```python
from build123d import *

# Parameters (mm, degrees)
SKETCH_1_R               = 11.5
EXTRUDE_1_DEPTH          = 10
SKETCH_2_R               = 13.945
EXTRUDE_2_DEPTH          = 13
SKETCH_3_R               = 16
EXTRUDE_3_DEPTH          = 1
EXTRUDE_START            = -1
SKETCH_4_R               = 16
EXTRUDE_4_DEPTH          = 1
CUT_EXTRUDE_1_DEPTH      = 33.26453161
CUT_EXTRUDE_1_DEPTH_BACK = 33.26453161
SKETCH_5_R               = 2.5


with BuildPart() as part:
    # 草图1 → 凸台-拉伸1 (new body)
    with BuildSketch(Plane.XY):
        Circle(SKETCH_1_R)
    extrude(amount=-EXTRUDE_1_DEPTH)

    # 草图2 → 凸台-拉伸2 (add)
    with BuildSketch(Plane(origin=(0, 0, -10), x_dir=(-1, 0, 0), z_dir=(0, 0, -1))):
        with Locations(Location((0, 0, 0), (0, 0, 180))):
            Circle(SKETCH_2_R)
    extrude(amount=EXTRUDE_2_DEPTH)

    # 草图3 → 凸台-拉伸3 (add)
    with BuildSketch(Plane(origin=(0, 0, -23), x_dir=(-1, 0, 0), z_dir=(0, 0, -1))):
        Circle(SKETCH_3_R)
    extrude(amount=-EXTRUDE_3_DEPTH)

    # 草图4 → 凸台-拉伸4 (add)
    with BuildSketch(Plane.XY.offset(-10).offset(EXTRUDE_START)):
        with Locations(Location((0, 0, 0), (0, 0, 180))):
            Circle(SKETCH_4_R)
    extrude(amount=EXTRUDE_4_DEPTH)

    # 草图5 → 切除-拉伸1 (cut, two sides: drawn at the far end of the back side and taken through both)
    with BuildSketch(Plane.XY.offset(-CUT_EXTRUDE_1_DEPTH_BACK)):
        Circle(SKETCH_5_R)
    extrude(amount=CUT_EXTRUDE_1_DEPTH + CUT_EXTRUDE_1_DEPTH_BACK, mode=Mode.SUBTRACT)


solid = part.part
```
The model under review builds one solid part; all positions refer to its coordinate system, in mm. A direction names the side the tool comes from. Coordinates: 2 decimals unless noted, no trailing zeros. Write each loop counter-clockwise with the first axis right and the second up, starting at its lowest first coordinate (ties: lowest second). Pieces come first, ordered by that corner, then holes. Notation, with made-up numbers: (-31, -30.75) -> (-14, -30.75) arc R30 cw to (-14, -4.75) -> close; hole circle Ø5 at (51, 58.5). An arc over 180 degrees is marked (long way). One line per item, written item: value. Start each with the question number.
Q1. Add section A-A, the plane y = 0. Give the boundary of the cut face in (x, z) (3 decimals).
Q2. Clearance check with flat-ended pins moving along their axes: P1, Ø2, axis at y = -10.5, z = -10.5, coming from the +X side; P2, Ø2, axis at y = 10, z = -19.5, coming from the -X side; P3, Ø1, axis at y = -10, z = -12, coming from the +X side. State where each tip first meets the part, or that it passes through.
Q3. The part is to be moulded in two halves that separate along Z. For faces 1 (the face through (0, 3, 0)), 2 (the face through (6.435, 12.372, -16.423)), 3 (the face through (-0.54, -2.44, -11.66)), 4 (the face through (-1.1, 14.3, -22)), say which applies: +Z half, -Z half, draft (parallel to the pull), parting line (faces both ways), or undercut.
Q4. For faces 5 (the face through (-1.5, 11.4, -4.9)), 6 (the face through (-3, 0, -23)), 7 (the face through (-1.1, -14.3, -11)), list the 3-axis set-ups (+Z, -Z, +X, -X, +Y, -Y) from which the entire face can be reached by the end or side of a thin tool; tool diameter is ignored.
Q5. To check wall thickness, follow probe 1 along Y at (x, z) = (0, -12.5) (3 decimals); probe 2 along Y at (x, z) = (0, -9.75); probe 3 along Z at (x, y) = (-14.5, 2.5). State the ranges of each line that lie inside material, in increasing order.
Q6. Add section D-D, the plane x = 8. Give the boundary of the cut face in (y, z), then the cut area to 3 significant figures.
Q7. Add section C-C, the plane z = -7.5. Give the boundary of the cut face in (x, y), then the cut area to 3 significant figures.
Response:
1. outline: (-16, -23) -> (-2.5, -23) -> (-2.5, 0) -> (-11.5, 0) -> (-11.5, -10) -> (-16, -10) -> (-16, -11) -> (-13.945, -11) -> (-13.945, -22) -> (-16, -22) -> close; (2.5, -23) -> (16, -23) -> (16, -22) -> (13.945, -22) -> (13.945, -11) -> (16, -11) -> (16, -10) -> (11.5, -10) -> (11.5, 0) -> (2.5, 0) -> close
2. P1: x = 12.87
2. P2: x = -10.65
2. P3: x = 10.21
3. face 1: +Z half
3. face 2: undercut
3. face 3: draft
3. face 4: undercut
4. face 5: +Z
4. face 6: -Z, +X, -X, +Y, -Y
4. face 7: none
5. probe 1: -13.945 to -2.5, 2.5 to 13.945
5. probe 2: -11.5 to -2.5, 2.5 to 11.5
5. probe 3: -23 to -22, -11 to -10
6. outline: (-13.86, -23) -> (13.86, -23) -> (13.86, -22) -> (11.42, -22) -> (11.42, -11) -> (13.86, -11) -> (13.86, -10) -> (8.26, -10) -> (8.26, 0) -> (-8.26, 0) -> (-8.26, -10) -> (-13.86, -10) -> (-13.86, -11) -> (-11.42, -11) -> (-11.42, -22) -> (-13.86, -22) -> close
6. area: 472 mm²
7. outline: circle Ø23 at (0, 0); hole circle Ø5 at (0, 0)
7. area: 396 mm²
